The model under review builds one solid part; all positions refer to its coordinate system, in mm. Face numbers are marked on the shaded views. A direction names the side the tool comes from. Give positions to 0.01 mm unless a question says otherwise; leave off trailing zeros. Loops run counter-clockwise (first coordinate to the right, second up) from the corner with the lowest first, then second, coordinate; pieces in that order, holes last. Notation, with made-up numbers: M -14,-30.5 L 0,-30.5 A24 cw 0,-18.5 Z; hole C -36,87 d8. An arc over 180 degrees is marked long. Return JSON: item names as keys, results as strings.
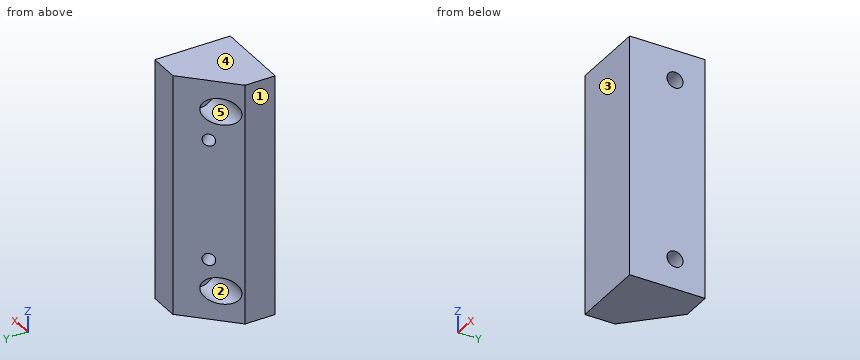
```python
from build123d import *

# Parameters (mm, degrees)
SKETCH1_W                                        = 31.75
SKETCH1_H                                        = 101.6
BOSS_EXTRUDE1_DEPTH                              = 15.875
CUT_EXTRUDE1_REACH                               = 106.051
F_1_4_20_TAPPED_HOLE1_D                          = 5.1054
F_1_4_20_TAPPED_HOLE1_DEPTH                      = 12.7
F_1_4_20_TAPPED_HOLE1_TIP                        = 1.533816902
CBORE_FOR_1_4_SOCKET_HEAD_CAP_SCREW1_D           = 6.7564
CBORE_FOR_1_4_SOCKET_HEAD_CAP_SCREW1_CBORE_D     = 11.1125
CBORE_FOR_1_4_SOCKET_HEAD_CAP_SCREW1_CBORE_DEPTH = 20.32


with BuildPart() as part:
    # Sketch1 → Boss-Extrude1 (new, symmetric)
    with BuildSketch(Plane(origin=(0, 0, 0), x_dir=(1, 0, 0), z_dir=(0, 1, 0))):
        Rectangle(SKETCH1_W, SKETCH1_H)
    extrude(amount=BOSS_EXTRUDE1_DEPTH, both=True)

    # Sketch2 → Cut-Extrude1 (cut, up to next)
    with BuildSketch(Plane.XY.offset(50.8), mode=Mode.PRIVATE) as cut_extrude1_sk1:
        Polygon((-15.875, -3.175), (-15.875, 15.875), (3.175, 15.875), align=None)
    cut_extrude1_tool1 = extrude(cut_extrude1_sk1.sketch, amount=-CUT_EXTRUDE1_REACH, mode=Mode.PRIVATE) & part.part
    add(cut_extrude1_tool1.solids().sort_by_distance((-9.525, 9.525, 50.8))[0], mode=Mode.SUBTRACT)

    # 1/4-20 Tapped Hole1
    with Locations(Plane(origin=(-6.35, 6.35, 0), x_dir=(0, 0, 1), z_dir=(-0.7071067811865513, 0.7071067811865438, 0))):
        with Locations((-25.4, 0), (25.4, 0)):
            Hole(F_1_4_20_TAPPED_HOLE1_D / 2, depth=F_1_4_20_TAPPED_HOLE1_DEPTH)
            with Locations((0, 0, -(F_1_4_20_TAPPED_HOLE1_DEPTH + F_1_4_20_TAPPED_HOLE1_TIP / 2))):  # 118° drill point
                Cone(0, F_1_4_20_TAPPED_HOLE1_D / 2, F_1_4_20_TAPPED_HOLE1_TIP, mode=Mode.SUBTRACT)

    # CBORE for 1/4 Socket Head Cap Screw1 (through all)
    with Locations(Plane.ZY.offset(15.875)):
        with Locations((-38.1, 3.175), (38.1, 3.175)):
            CounterBoreHole(CBORE_FOR_1_4_SOCKET_HEAD_CAP_SCREW1_D / 2, CBORE_FOR_1_4_SOCKET_HEAD_CAP_SCREW1_CBORE_D / 2, CBORE_FOR_1_4_SOCKET_HEAD_CAP_SCREW1_CBORE_DEPTH)


solid = part.part
```
1) Consider section B-B on z = 40. Write out the cut boundary in (x, y) (3 decimals), then the cut area to 3 significant figures.
From the geometry:
{"outline": "M -15.875,-15.875 L 15.875,-15.875 L 15.875,0.382 L 4.445,0.382 L 4.445,-2.046 L -14.746,-2.046 L -15.875,-3.175 Z; M -4.304,8.396 L 4.445,8.396 L 4.445,5.968 L 15.875,5.968 L 15.875,15.875 L 3.175,15.875 Z", "area": "617 mm²"}
2) Wall thickness on L1, parallel to Z at x = -9, y = 3.5; L2, parallel to Z at x = -6, y = 4; L3, parallel to Z at x = 10, y = 1: over which ranges is each line inside the solid? List them lowest first. Write a range as from..to.
From the geometry:
{"L1": "-50.8..-43.65, -32.55..32.55, 43.65..50.8", "L2": "-50.8..-43.59, -32.61..-27.53, -23.27..23.27, 27.53..32.61, 43.59..50.8", "L3": "-50.8..-40.68, -35.52..35.52, 40.68..50.8"}
3) Insertion check: pin 1 (9 mm diameter, centred on y = 1.5, z = 38, fed in from -X); pin 2 (8 mm diameter, centred on y = 3.175, z = 38.1, fed in from -X) (3 decimals). Each pin has a flat end and moves straight along its axis. Give the tip position at first contact, or say it passes through.
From the geometry:
{"pin 1": "x = -15.7", "pin 2": "x = 4.445"}
4) Consider section D-D on x = -14. Write out the cut boundary in (y, z) (1 decimal).
From the geometry:
{"outline": "M -15.9,-50.8 L -1.3,-50.8 L -1.3,-41.4 A5.6 cw -1.3,-34.8 L -1.3,34.8 A5.6 cw -1.3,41.4 L -1.3,50.8 L -15.9,50.8 Z"}
5) The part is to be moulded in two halves that separate along Y. For the marked faces 1, 2 and 3, say which applies: released by +Y, released by -Y, zero draft, split by the parting line, or undercut.
From the geometry:
{"face 1": "zero draft", "face 2": "undercut", "face 3": "released by -Y"}
6) Consider section C-C on z = 6.5. Write out the cut boundary in (x, y) (3 decimals), then the cut area to 3 significant figures.
From the geometry:
{"outline": "M -15.875,-15.875 L 15.875,-15.875 L 15.875,15.875 L 3.175,15.875 L -15.875,-3.175 Z", "area": "827 mm²"}
7) Tool access review of the marked faces 4 and 5: name each direction out of +Z, -Z, +X, -X, +Y, -Y from which nothing blocks a thin tool from reaching the whole face with its end or side.
From the geometry:
{"face 4": "+Z, +X, -X, +Y, -Y", "face 5": "-X"}
8) Consider section A-A on x = 8. Write out the cut boundary in (y, z) (3 decimals), then the cut area to 3 significant figures.
From the geometry:
{"outline": "M -15.875,-50.8 L 15.875,-50.8 L 15.875,50.8 L -15.875,50.8 Z; hole C 3.175,-38.1 d6.756; hole C 3.175,38.1 d6.756", "area": "3,150 mm²"}
